Read the model definition and answer for the solid it produces. Units are mm, in the model's axes. A direction names the side the tool comes from. Give positions to 0.01 mm unless a question says otherwise; leave off trailing zeros. Order: outer loops, then holes, each group sorted by start corner. A loop starts at its lowest first (then second) coordinate and runs counter-clockwise, first axis right, second up. Notation, with made-up numbers: M 41.5,53 L 91.5,53 A19 ccw 91.5,76 Z; hole C 60,73 d10. An arc over 180 degrees is marked long. Write item = value, one per line. Start each with the question number.
from build123d import *

# Parameters (mm, degrees)
SKETCH1_R               = 4
BOSS_EXTRUDE1_DEPTH     = 39.5
SKETCH2_W               = 25
SKETCH2_H               = 75.25
CUT_EXTRUDE1_DEPTH      = 105.5
CUT_EXTRUDE1_DEPTH_BACK = 117.5
CUT_EXTRUDE2_DEPTH      = 43.5
SKETCH4_R               = 6
CUT_EXTRUDE3_DEPTH      = 41


with BuildPart() as part:
    # Sketch1 → Boss-Extrude1 (new body)
    with BuildSketch(Plane(origin=(0, 0, 0), x_dir=(0, 0, -1), z_dir=(1, 0, 0))):
        with BuildLine():
            Line((0, -40), (0, 40))
            Line((0, 40), (25, 40))
            Line((25, 40), (73.280107592, 70.785366831))
            ThreePointArc((73.280107592, 70.785366831), (80.81695996, 72.117470486), (87.088258906, 67.730050596))
            Line((87.088258906, 67.730050596), (103.222887942, 42.426417539))
            ThreePointArc((103.222887942, 42.426417539), (104.391084837, 39.850237691), (104.791154167, 37.05))
            Line((104.791154167, 37.05), (104.791154167, -37.05))
            ThreePointArc((104.791154167, -37.05), (104.391084837, -39.850237691), (103.222887942, -42.426417539))
            Line((103.222887942, -42.426417539), (87.088258906, -67.730050596))
            ThreePointArc((87.088258906, -67.730050596), (80.81695996, -72.117470486), (73.280107592, -70.785366831))
            Line((73.280107592, -70.785366831), (25, -40))
            Line((25, -40), (0, -40))
        make_face()
        with Locations((78.7, 62.25)):
            Circle(SKETCH1_R, mode=Mode.SUBTRACT)
        with Locations((95, 37.153633057)):
            Circle(SKETCH1_R, mode=Mode.SUBTRACT)
        with Locations((95, -37.153633057)):
            Circle(SKETCH1_R, mode=Mode.SUBTRACT)
        with Locations((78.7, -62.25)):
            Circle(SKETCH1_R, mode=Mode.SUBTRACT)
        Polygon((30.81, -20), (30.81, 20), (75.651092334, 48.552793879), (84.857166207, 34.095), (84.857166207, -34.095), (75.651092334, -48.552793879), align=None, mode=Mode.SUBTRACT)
    extrude(amount=BOSS_EXTRUDE1_DEPTH)

    # Sketch2 → Cut-Extrude1 (cut, two sides)
    with BuildSketch(Plane(origin=(0, 0, 0), x_dir=(1, 0, 0), z_dir=(0, 1, 0))) as cut_extrude1_sk:
        with Locations((19.75, 57.625)):
            Rectangle(SKETCH2_W, SKETCH2_H)
    extrude(amount=CUT_EXTRUDE1_DEPTH, mode=Mode.SUBTRACT)
    extrude(cut_extrude1_sk.sketch, amount=-CUT_EXTRUDE1_DEPTH_BACK, mode=Mode.SUBTRACT)

    # Sketch3 → Cut-Extrude2 (cut)
    with BuildSketch(Plane(origin=(0, 0, -104.791154167), x_dir=(-1, 0, 0), z_dir=(0, 0, -1))):
        Polygon((-7.25, -37.05), (-7.25, -12.5), (-32.25, -12.5), (-32.25, -37.05), (-32.25, -54.930146657), (-7.25, -54.930146657), align=None)
        Polygon((-32.25, 37.05), (-32.25, 12.5), (-7.25, 12.5), (-7.25, 37.05), (-7.25, 54.930146657), (-32.25, 54.930146657), align=None)
    extrude(amount=-CUT_EXTRUDE2_DEPTH, mode=Mode.SUBTRACT)

    # Sketch4 → Cut-Extrude3 (cut)
    with BuildSketch(Plane.XY):
        with Locations((19.75, 0)):
            Circle(SKETCH4_R)
    extrude(amount=-CUT_EXTRUDE3_DEPTH, mode=Mode.SUBTRACT)


solid = part.part
1) Find section C-C on y = 0. Determine the outline of the cut face in (x, z), plus the area to 3 significant figures.
2) Each of these flat-tipped pins is pushed along its axis until it touches: P1, Ø7.5, axis at x = 21.5, z = -99, coming from the -Y side; P2, Ø9.5, axis at x = 19.75, y = 0, coming from the +Z side; P3, Ø1.5, axis at x = 33.5, z = -52.5, coming from the +Y side; P4, Ø6.5, axis at y = -37.15, z = -95, coming from the -X side. Where does it stop, or does it pass through?
3) For a pull along Y with two mould halves and no side action, classify faces 4 (the face through (35.82, -55.61, -49.48)), 5 (the face through (25.29, -2.3, -9.86)), 6 (the face through (3.574, 55.177, -48.802)) as pulls with the +Y half, pulls with the -Y half, needs draft (parallel to the pull), parting line crosses it, or undercut.
4) For faces 1 (the face through (20, 12.5, -100)), 2 (the face through (3.57, -54.9, -95.27)), 3 (the face through (3.574, -34.476, -53.544)), determine the directions among +Z, -Z, +X, -X, +Y, -Y from which every point of the face is accessible in a straight line to the end or side of a thin tool.
5) Find section B-B on x = 30. Determine the outline of the cut face in (y, z).
6) Find the intervals of material crossed by probe 1 along Y at (x, z) = (4.5, -95); probe 2 along X at (y, z) = (-20.5, -22); probe 3 along Y at (x, z) = (6, -92.5), in increasing order. Write a range as [from, to].
7) Find section D-D on z = -78.7. Count the separate pieces of the cut face and the enclosed holes in it, plus the area to 3 significant figures.
8) Find section A-A on z = -7.5. Determine the outline of the cut face in (x, y), plus the area to 3 significant figures.
Numbers:
q1.outline = M 0,-104.79 L 39.5,-104.79 L 39.5,-84.86 L 32.25,-84.86 L 32.25,-95.25 L 7.25,-95.25 L 7.25,-84.86 L 0,-84.86 Z; M 0,-30.81 L 7.25,-30.81 L 7.25,-20 L 13.75,-20 L 13.75,0 L 0,0 Z; M 25.75,-20 L 32.25,-20 L 32.25,-30.81 L 39.5,-30.81 L 39.5,0 L 25.75,0 Z
q1.area = 1,230 mm2
q2.P1 = -12.5
q2.P2 = -95.25
q2.P3 = 58.01
q2.P4 = through
q3.face_4 = pulls with the -Y half
q3.face_5 = undercut
q3.face_6 = pulls with the +Y half
q4.face_1 = -Z, +Y
q4.face_2 = -Z, +X, -X, -Y
q4.face_3 = +X, -X
q5.outline = M -40,-20 L 40,-20 L 40,0 L -40,0 Z; M -12.5,-104.79 L 12.5,-104.79 L 12.5,-95.25 L -12.5,-95.25 Z
q6.probe_1 = [-55.32, -41.15], [-33.15, 33.15], [41.15, 55.32]
q6.probe_2 = [0, 7.25], [32.25, 39.5]
q6.probe_3 = [-59.24, -40.28], [-34.03, 34.03], [40.28, 59.24]
q7.separate_pieces = 8
q7.enclosed_holes = 0
q7.area = 597 mm2
q8.outline = M 0,-40 L 39.5,-40 L 39.5,40 L 0,40 Z; hole C 19.75,0 d12
q8.area = 3,050 mm2
